from build123d import *

# Parameters (mm, degrees)
BOSS_EXTRU_2_DEPTH = 5
BOSS_EXTRU_3_DEPTH = 50
ESQUISSE3_W        = 65
ESQUISSE3_H        = 200
BOSS_EXTRU_7_DEPTH = 5
ESQUISSE8_W        = 65
ESQUISSE8_H        = 200
BOSS_EXTRU_8_DEPTH = 5


with BuildPart() as part:
    # Esquisse1 → Boss.-Extru.2 (new body)
    with BuildSketch(Plane.XY):
        Polygon((-50, 100), (-110, 100), (-110, 150), (-50, 150), (-50, 200), (0, 200), (0, 150), (60, 150), (60, 100), (0, 100), (0, 0), (-50, 0), align=None)
    extrude(amount=BOSS_EXTRU_2_DEPTH)

    # Esquisse2 → Boss.-Extru.3 (add)
    with BuildSketch(Plane.XY.offset(5)):
        Polygon((-110, 150), (-110, 100), (-50, 100), (-50, 0), (0, 0), (0, 100), (60, 100), (60, 150), (0, 150), (0, 200), (-50, 200), (-50, 150), align=None)
        Polygon((-105, 145), (-105, 105), (-45, 105), (-45, 5), (-5, 5), (-5, 105), (55, 105), (55, 145), (-5, 145), (-5, 195), (-45, 195), (-45, 145), align=None, mode=Mode.SUBTRACT)
    extrude(amount=BOSS_EXTRU_3_DEPTH)

    # Esquisse3 → Boss.-Extru.7 (add)
    with BuildSketch(Plane.XY.offset(55)):
        with Locations((-77.636000324, 100)):
            Rectangle(ESQUISSE3_W, ESQUISSE3_H)
    extrude(amount=BOSS_EXTRU_7_DEPTH)

    # Esquisse8 → Boss.-Extru.8 (add)
    with BuildSketch(Plane.XY.offset(55)):
        with Locations((28.350884712, 100)):
            Rectangle(ESQUISSE8_W, ESQUISSE8_H)
    extrude(amount=BOSS_EXTRU_8_DEPTH)


solid = part.part
Source: CAD feature listing. Evaluate the final solid. Frame: model axes, mm. A direction names the side the tool comes from. Round coordinates to 2 decimals unless told otherwise and drop trailing zeros. Write each loop counter-clockwise with the first axis right and the second up, starting at its lowest first coordinate (ties: lowest second). Pieces come first, ordered by that corner, then holes. Notation, with made-up numbers: M -25.75,0 L 26.25,0 A27 cw 26.25,17 Z; hole C 41,42.5 d6. An arc over 180 degrees is marked long. One line per item, written item: value. Start each with the question number.
Item 1: Section query C-C (y = 64.5). Return the cut outline in (x, z), plus the area to 3 significant figures.
Item 2: Section query A-A (z = 14.5). Return the cut outline in (x, y), plus the area to 3 significant figures.
Item 3: Ray query, L1, parallel to Y at x = 50, z = 23.5; L2, parallel to X at y = 18, z = 5.5; L3, parallel to X at y = 142, z = 6. Return the intervals inside material, ascending. Write a range as from..to.
Item 4: Set-up query: faces 1 (the flat face through (-24, 101, 5)), 2 (the flat face through (-45, 56, 30)), 3 (the flat face through (-25, 2, 55)), 4 (the flat face through (30, 150, 27)). Return all of +Z, -Z, +X, -X, +Y, -Y with unobstructed straight access to the full face (end or side cutting, diameter ignored); none if empty.
Item 5: Section query B-B (x = -86). Return the cut outline in (y, z).
Item 6: Mould query, pull axis X, two halves, no side actions, for faces 5 (the flat face through (30, 100, 27)), 6 (the flat face through (-50, 175, 27)), 7 (the flat face through (-105, 125, 30)), 8 (the flat face through (0, 175, 27)). Classes: pulls with the +X half, pulls with the -X half, needs draft (parallel to the pull), parting line crosses it, or undercut.
Item 7: Section query D-D (x = -42). Return the cut outline in (y, z), plus the area to 3 significant figures.
Item 8: Pin query (flat end, axial travel): pin 1 (2 mm diameter, centred on x = -12.5, z = 20.5, fed in from -Y); pin 2 (8 mm diameter, centred on y = 126.5, z = 23.5, fed in from -X); pin 3 (1 mm diameter, centred on y = 156, z = 28, fed in from -X); pin 4 (15 mm diameter, centred on x = -84, z = 26.5, fed in from +Y). Return the tip coordinate at first contact, or that it passes through.
Result set:
1. outline: M -110.14,55 L -50,55 L -50,0 L 0,0 L 0,55 L 60.85,55 L 60.85,60 L -4.15,60 L -4.15,55 L -5,55 L -5,5 L -45,5 L -45,55 L -45.14,55 L -45.14,60 L -110.14,60 Z
1. area: 1,400 mm²
2. outline: M -110,100 L -50,100 L -50,0 L 0,0 L 0,100 L 60,100 L 60,150 L 0,150 L 0,200 L -50,200 L -50,150 L -110,150 Z; hole M -105,105 L -45,105 L -45,5 L -5,5 L -5,105 L 55,105 L 55,145 L -5,145 L -5,195 L -45,195 L -45,145 L -105,145 Z
2. area: 3,600 mm²
3. L1: y = 100..105, 145..150
3. L2: x = -50..-45, -5..0
3. L3: x = -110..-105, 55..60
4. face 1: none
4. face 2: +Z
4. face 3: +Z, +Y, -Y
4. face 4: -Z, +X, +Y
5. outline: M 0,55 L 100,55 L 100,0 L 150,0 L 150,55 L 200,55 L 200,60 L 0,60 Z; hole M 105,5 L 145,5 L 145,55 L 105,55 Z
6. face 5: needs draft
6. face 6: pulls with the -X half
6. face 7: undercut
6. face 8: pulls with the +X half
7. outline: M 0,0 L 200,0 L 200,55 L 195,55 L 195,5 L 5,5 L 5,55 L 0,55 Z
7. area: 1,500 mm²
8. pin 1: stops at y = 0
8. pin 2: stops at x = -110
8. pin 3: stops at x = -50
8. pin 4: stops at y = 150
